Here's how the part is built. I have some questions about the finished solid (model axes, mm). A direction names the side the tool comes from. Round coordinates to 2 decimals unless told otherwise and drop trailing zeros. Loops run counter-clockwise (first coordinate to the right, second up) from the corner with the lowest first, then second, coordinate; pieces in that order, holes last. Notation, with made-up numbers: M 44.25,16 L 82.25,16 A7 ccw 82.25,29 Z; hole C -19.75,22 d9. An arc over 180 degrees is marked long. Answer as a JSON object with one key per item and string values.
Autodesk Inventor part; units mm, degrees
ref_plane "Work Plane2" through (0, 12.5, 0) normal (0, 1, 0) x (-1, 0, 0)
ref_plane "YZ Plane" through (0, 0, 0) normal (1, 0, 0) x (0, 1, 0)
ref_plane "XY Plane" through (0, 0, 0) normal (0, 0, 1) x (1, 0, 0)
sketch "Sketch1" plane through (0, 0, 0) normal (0, 0, 1) x (1, 0, 0)
  circle A0 centre (0, 0) radius 7.5
  circle A1 centre (0, 0) radius 12.5
  dimension "d0" = 15
  dimension "d1" = 25
extrude "Extrusion1" add sketch "Sketch1" along normal blind 698
ref_plane "Work Plane2" through (0, 12.5, 0) normal (0, 1, 0) x (-1, 0, 0)
sketch "Sketch3" plane through (0, 12.5, 0) normal (0, 1, 0) x (-1, 0, 0)
  line L0 (219.2482, 398) -> (-262.0284, 398)
  line L1 (12.5, 698) -> (-12.5, 698)
  line L2 (351.4203, 300) -> (-288.0764, 300)
  line L3 (12.5, 0) -> (-12.5, 0)
  point P0 (0, 0)
  dimension "d7" = 300
  dimension "d8" = 300
bend part "Bend Part1" radius 12.7 angle 90 line through (-219.2482, 12.5, 398) along (1, 0, 0) centre toward (0, 1, 0) moving side (0, 0, 1) both sides no
sketch "Sketch4" plane through (0, 12.5, 0) normal (0, 1, 0) x (-1, 0, 0)
  line L0 (312.7899, 300) -> (-276.8847, 300)
  line L1 (12.5, 0) -> (-12.5, 0)
  point P0 (0, 0)
  dimension "d11" = 300
bend part "Bend Part2" radius 12.7 angle 90 line through (-312.7899, 12.5, 300) along (1, 0, 0) centre toward (0, 1, 0) moving side (0, 0, -1) both sides no
sketch "Sketch5" plane through (0, 305.2509, 423.2) normal (0, 1, 0) x (1, 0, 0)
  point P0 (0, 423.2)
properties part number "Seat Link"
Item 1: I'm going to push flat-ended pins straight in: pin 1 Ø1.5 at (x, y) = (-6.5, 245) entering from +Z; pin 2 Ø1.5 at (x, z) = (3, 322.5) entering from +Y; pin 3 Ø12 at (x, z) = (-8, 399.5) entering from -Y. Where does each tip first touch, or does it pass through?
Resolved:
{"pin 1": "z = 434.3", "pin 2": "y = 12.3", "pin 3": "y = -12.32"}
Item 2: I want a section at C-C, the plane z = 340. Please give me the cut outline in (x, y), then the cut area to 3 significant figures.
Resolved:
{"outline": "C 0,0 d25; hole C 0,0 d15", "area": "314 mm²"}
Item 3: If we mould it in two halves opening along Z, with no side actions, what happens to faces 1 (the face through (5, 305.251, 429)), 2 (the face through (-1.627, 167.186, 262.406)), 3 (the face through (-7.493, -0.33, 348.314))? For each: pulls with the +Z half, pulls with the -Z half, needs draft (parallel to the pull), parting line crosses it, or undercut.
Resolved:
{"face 1": "needs draft", "face 2": "undercut", "face 3": "undercut"}
Item 4: I want a section at A-A, the plane x = 0. Please give me the cut outline in (y, z), then the cut area to 3 significant figures.
Resolved:
{"outline": "M -12.5,300 A37.7 ccw 25.2,262.3 L 305.25,262.3 L 305.25,267.3 L 25.2,267.3 A32.7 cw -7.5,300 L -7.5,398 A32.7 cw 25.2,430.7 L 305.25,430.7 L 305.25,435.7 L 25.2,435.7 A37.7 ccw -12.5,398 Z; M 7.5,300 A17.7 ccw 25.2,282.3 L 305.25,282.3 L 305.25,287.3 L 25.2,287.3 A12.7 cw 12.5,300 L 12.5,398 A12.7 cw 25.2,410.7 L 305.25,410.7 L 305.25,415.7 L 25.2,415.7 A17.7 ccw 7.5,398 Z", "area": "7,370 mm²"}
Item 5: Please list where these lines run through material, in increasing order: probe 1 along Z at (x, y) = (-1, 208); probe 2 along Z at (x, y) = (0, 221.5); probe 3 along Y at (x, z) = (0, 326.5). Write a range as from..to.
Resolved:
{"probe 1": "262.34..267.37, 282.23..287.26, 410.74..415.77, 430.63..435.66", "probe 2": "262.3..267.3, 282.3..287.3, 410.7..415.7, 430.7..435.7", "probe 3": "-12.5..-7.5, 7.5..12.5"}
Item 6: On a 3-axis mill with a long thin cutter (end or side, diameter ignored), from which of +Z, -Z, +X, -X, +Y, -Y can I reach the whole of each face in a straight line? I mean faces 4 (the face through (5, 305.251, 269)), 5 (the face through (11.923, -3.755, 348.314)), 6 (the face through (-0.976, 167.186, 267.364)). Say none if no direction works.
Resolved:
{"face 4": "+Z, -Z, +X, -X, +Y", "face 5": "none", "face 6": "+Y"}
Item 7: I want a section at B-B, the plane y = 104.5. Please give me the cut outline in (x, z).
Resolved:
{"outline": "C 0,274.8 d25; C 0,423.2 d25; hole C 0,274.8 d15; hole C 0,423.2 d15"}
